from build123d import *

# Parameters (mm, degrees)
F3_D     = 6.35
F4_R     = 5.5
F5_DEPTH = 7.5
F7_D     = 6.35


with BuildPart() as f1:
    # F0 (on Right) → F1 (revolve)
    with BuildSketch(Plane.YZ):
        Polygon((0, 37.062926), (0, -35.937074), (6, -35.937074), (6, 15.529456), (5, 15.529456), (5, 26.525273), (15, 26.525273), (15, 29.579665), (7, 29.579665), (7, 37.062926), align=None)
    revolve(axis=Axis((0, 0, 0.562926), (0, 0, 1)))

    # F3 (through all)
    with Locations(Plane.XY.offset(37.062926)):
        with Locations((0, 0)):
            Hole(F3_D / 2)

    # F4 (on Right) → F5 (join, symmetric)
    with BuildSketch(Plane.YZ):
        with Locations((0, 2.529456)):
            Circle(F4_R)
    extrude(amount=F5_DEPTH, both=True)

    # F7 (through all)
    with Locations(Plane.YZ.offset(7.5)):
        with Locations((0, 2.529456)):
            Hole(F7_D / 2)


solid = f1.part
Input: part model. Units: mm. Frame: model coordinates. A direction names the side the tool comes from. Round coordinates to 2 decimals unless told otherwise and drop trailing zeros. Loops run counter-clockwise (first coordinate to the right, second up) from the corner with the lowest first, then second, coordinate; pieces in that order, holes last. Notation, with made-up numbers: (-1, 22) -> (26, 22) arc R5 cw to (26, 31) -> close; hole circle Ø8 at (63, -10). An arc over 180 degrees is marked (long way). Answer as a JSON object with one key per item and string values. Group by question number.
1) Section query D-D on x = -12.25. Output: boundary loops of the cut face in (y, z).
2) Section query B-B on x = 0. Output: boundary loops of the cut face in (y, z) (3 decimals).
3) Section query A-A on z = 4.5. Output: boundary loops of the cut face in (x, y).
4) Draft query along Y for faces 1 (the cylindrical face through (2.681, 6.466, 33.374)), 2 (the cylindrical face through (0.69, -3.1, -19.19)), 3 (the flat face through (3, 1.5, 37.063)). Return one class per face: +Y half, -Y half, draft (parallel to the pull), parting line (faces both ways), or undercut.
5) Ray query, L1, parallel to X at y = 0, z = 19 (3 decimals); L2, parallel to X at y = 0, z = 14.5 (3 decimals). Return the intervals inside material, ascending.
6) Reachability of faces 4 (the flat face through (-7.5, 2.4, 0.2)), 5 (the flat face through (-4, -4, 15.529)), 6 (the cylindrical face through (5.55, 5.08, 0.42)), 7 (the cylindrical face through (-5.48, 5.08, 0.42)) from +Z, -Z, +X, -X, +Y, -Y: full face, straight path, thin tool, end or side. Return the list, or none.
7) Section query C-C on z = -4. Output: boundary loops of the cut face in (x, y) (3 decimals), plus the area to 3 significant figures.
8) Pin query (flat end, axial travel): pin 1 (1.5 mm diameter, centred on x = -1.5, y = -10.5, fed in from -Z); pin 2 (3.5 mm diameter, centred on y = 2.5, z = 3, fed in from -X); pin 3 (5.5 mm diameter, centred on y = -2, z = 3.5, fed in from +X). Return the tip coordinate at first contact, or that it passes through.
Reply:
{
 "1": {"outline": "(-8.66, 26.53) -> (8.66, 26.53) -> (8.66, 29.58) -> (-8.66, 29.58) -> close"},
 "2": {"outline": "(-15, 26.525) -> (-5, 26.525) -> (-5, 15.529) -> (-6, 15.529) -> (-6, -35.937) -> (-3.175, -35.937) -> (-3.175, -1.962) arc R5.5 ccw to (3.175, -1.962) -> (3.175, -35.937) -> (6, -35.937) -> (6, 15.529) -> (5, 15.529) -> (5, 26.525) -> (15, 26.525) -> (15, 29.58) -> (7, 29.58) -> (7, 37.063) -> (3.175, 37.063) -> (3.175, 7.02) arc R5.5 ccw to (-3.175, 7.02) -> (-3.175, 37.063) -> (-7, 37.063) -> (-7, 29.58) -> (-15, 29.58) -> close; hole circle Ø6.35 at (0, 2.529)"},
 "3": {"outline": "(-7.5, -5.13) -> (-3.1, -5.13) arc R6 ccw to (3.1, -5.13) -> (7.5, -5.13) -> (7.5, -2.49) -> (-7.5, -2.49) -> close; (-7.5, 2.49) -> (7.5, 2.49) -> (7.5, 5.13) -> (3.1, 5.13) arc R6 ccw to (-3.1, 5.13) -> (-7.5, 5.13) -> close"},
 "4": {"face 1": "parting line", "face 2": "undercut", "face 3": "draft"},
 "5": {"L1": "x = -5 to -3.175, 3.175 to 5", "L2": "x = -6 to -3.175, 3.175 to 6"},
 "6": {"face 4": "-Z, -X, +Y, -Y", "face 5": "none", "face 6": "+X", "face 7": "-X"},
 "7": {"outline": "circle Ø12 at (0, 0); hole circle Ø6.35 at (0, 0)", "area": "81.4 mm2"},
 "8": {"pin 1": "stops at z = 26.53", "pin 2": "stops at x = -7.5", "pin 3": "stops at x = 7.5"}
}
